```python
from build123d import *

# Parameters (mm, degrees)
BOSS_EXTRUDE1_DEPTH = 5.588
SKETCH2_W           = 6.096
SKETCH2_H           = 12.7
CUT_EXTRUDE1_DEPTH  = 5.588


with BuildPart() as part:
    # Sketch1 → Boss-Extrude1 (new body)
    with BuildSketch(Plane(origin=(0, 0, 0), x_dir=(1, 0, 0), z_dir=(0, 1, 0))):
        Polygon((-108.712, 6.35), (-114.3, 6.35), (-114.3, -6.35), (-108.712, -6.35), (-108.712, -60.325), (-38.862, -60.325), (-38.862, -65.913), (-26.162, -65.913), (-26.162, -60.325), (26.162, -60.325), (26.162, -65.913), (38.862, -65.913), (38.862, -60.325), (108.712, -60.325), (108.712, -6.35), (114.3, -6.35), (114.3, 6.35), (108.712, 6.35), (108.712, 60.325), (38.862, 60.325), (38.862, 65.913), (26.162, 65.913), (26.162, 60.325), (-26.162, 60.325), (-26.162, 65.913), (-38.862, 65.913), (-38.862, 60.325), (-108.712, 60.325), align=None)
    extrude(amount=BOSS_EXTRUDE1_DEPTH)

    # Sketch2 → Cut-Extrude1 (cut)
    with BuildSketch(Plane.XZ):
        with Locations((-34.544, 31.623)):
            Rectangle(SKETCH2_W, SKETCH2_H)
        with Locations((98.044, 31.623)):
            Rectangle(SKETCH2_W, SKETCH2_H)
        with Locations((98.044, -31.623)):
            Rectangle(SKETCH2_W, SKETCH2_H)
        with Locations((-34.544, -31.623)):
            Rectangle(SKETCH2_W, SKETCH2_H)
    extrude(amount=-CUT_EXTRUDE1_DEPTH, mode=Mode.SUBTRACT)


solid = part.part
```
Can you work these out from the model? Positions are in its coordinate system, mm. A direction names the side the tool comes from. Coordinates: 2 decimals unless noted, no trailing zeros. Write each loop counter-clockwise with the first axis right and the second up, starting at its lowest first coordinate (ties: lowest second). Pieces come first, ordered by that corner, then holes. Notation, with made-up numbers: (16.5, 37.5) - (63.5, 37.5) arc R20 cw to (63.5, 57.5) - close; hole circle Ø10 at (20, 39). An arc over 180 degrees is marked (long way). Return JSON: item names as keys, results as strings.
Q1. I'm going to push flat-ended pins straight in: pin 1 Ø3 at (y, z) = (1.5, 33) entering from +X; pin 2 Ø1.5 at (y, z) = (4.5, -22) entering from -X; pin 3 Ø3 at (x, y) = (-88, 2) entering from +Z (3 decimals). Where does each tip first touch, or does it pass through?
Computed values:
{"pin 1": "stops at x = 108.71", "pin 2": "stops at x = -108.71", "pin 3": "stops at z = 60.325"}
Q2. Thinking about a two-plate mould opening in X: for faces 5 (the flat face through (-35, 3, 25.273)), 6 (the flat face through (38.862, 3, -63)), 7 (the flat face through (32, 3, 65.913)), which applies, +X half, -X half, draft (parallel to the pull), parting line (faces both ways), or undercut?
Computed values:
{"face 5": "undercut", "face 6": "+X half", "face 7": "draft"}
Q3. On a 3-axis mill with a long thin cutter (end or side, diameter ignored), from which of +Z, -Z, +X, -X, +Y, -Y can I reach the whole of each face in a straight line? I mean faces 1 (the flat face through (0, 3, 60.325)), 2 (the flat face through (111, 3, 6.35)), 3 (the flat face through (-74, 3, 60.325)), 4 (the flat face through (98, 3, 37.973)). Say none if no direction works.
Computed values:
{"face 1": "+Z, +Y, -Y", "face 2": "+Z, +X, +Y, -Y", "face 3": "+Z, -X, +Y, -Y", "face 4": "+Y, -Y"}
Q4. Please list where these lines run through material, in increasing order: L1, parallel to X at y = 2.5, z = -34; L2, parallel to Z at x = -45, y = 2.1 (3 decimals); L3, parallel to X at y = 0.95, z = 7. Write a range as from..to.
Computed values:
{"L1": "x = -108.71..-37.59, -31.5..95, 101.09..108.71", "L2": "z = -60.325..60.325", "L3": "x = -108.71..108.71"}
Q5. If we section it at D-D (z = 11): Please give me the cut outline in (x, y).
Computed values:
{"outline": "(-108.71, 0) - (108.71, 0) - (108.71, 5.59) - (-108.71, 5.59) - close"}
Q6. If we section it at B-B (x = -78): Please give me the cut outline in (y, z) (3 decimals), then the cut area to 3 significant figures.
Computed values:
{"outline": "(0, -60.325) - (5.588, -60.325) - (5.588, 60.325) - (0, 60.325) - close", "area": "674 mm2"}
Q7. If we section it at A-A (z = -32): Please give me the cut outline in (x, y), then the cut area to 3 significant figures.
Computed values:
{"outline": "(-108.71, 0) - (-37.59, 0) - (-37.59, 5.59) - (-108.71, 5.59) - close; (-31.5, 0) - (95, 0) - (95, 5.59) - (-31.5, 5.59) - close; (101.09, 0) - (108.71, 0) - (108.71, 5.59) - (101.09, 5.59) - close", "area": "1,150 mm2"}
Q8. If we section it at C-C (y = 1.2): Count the separate pieces of the cut face and the enclosed holes in it, then the cut area to 3 significant figures.
Computed values:
{"separate pieces": "1", "enclosed holes": "4", "area": "26,300 mm2"}
